```python
from build123d import *

# Parameters (mm, degrees)
SKETCH_1_W          = 72
SKETCH_1_H          = 16
SKETCH_1_R          = 3.1
EXTRUDE_1_DEPTH     = 4
EXTRUDE_START       = -4
SKETCH_3_W          = 30
SKETCH_3_H          = 5
EXTRUDE_2_DEPTH     = 60
SKETCH_5_W          = 108
SKETCH_5_H          = 11
SKETCH_5_R          = 2.1
EXTRUDE_3_DEPTH     = 5
SKETCH_6_W          = 12
SKETCH_6_H          = 11
CUT_EXTRUDE_1_DEPTH = 2
SKETCH_7_W          = 15
SKETCH_7_H          = 50
CUT_EXTRUDE_2_DEPTH = 86.599357474
EXTRUDE_4_DEPTH     = 2
EXTRUDE_START_2     = -30
EXTRUDE_5_DEPTH     = 2
FILLET_1_R          = 2


with BuildPart() as part:
    # 草图1 → 凸台-拉伸1 (new body)
    with BuildSketch(Plane.XY):
        Rectangle(SKETCH_1_W, SKETCH_1_H)
        with Locations((-27.5, 0)):
            Circle(SKETCH_1_R, mode=Mode.SUBTRACT)
        with Locations(Location((27.5, 0, 0), (0, 0, 180))):
            Circle(SKETCH_1_R, mode=Mode.SUBTRACT)
    extrude(amount=EXTRUDE_1_DEPTH)

    # 草图3 → 凸台-拉伸2 (add)
    with BuildSketch(Plane.XY.offset(4).offset(EXTRUDE_START)):
        with Locations((0, -5.5)):
            Rectangle(SKETCH_3_W, SKETCH_3_H)
    extrude(amount=EXTRUDE_2_DEPTH)

    # 草图5 → 凸台-拉伸3 (add, through all)
    with BuildSketch(Plane(origin=(0, -3, 0), x_dir=(1, 0, 0), z_dir=(0, 1, 0))):
        with Locations((0, -60)):
            Rectangle(SKETCH_5_W, SKETCH_5_H)
        with Locations(Location((47.5, -60, 0), (0, 0, 270))):
            Circle(SKETCH_5_R, mode=Mode.SUBTRACT)
        with Locations(Location((-47.5, -60, 0), (0, 0, 90))):
            Circle(SKETCH_5_R, mode=Mode.SUBTRACT)
    extrude(amount=-EXTRUDE_3_DEPTH)

    # 草图6 → 切除-拉伸1 (cut)
    with BuildSketch(Plane(origin=(0, -3, 0), x_dir=(1, 0, 0), z_dir=(0, 1, 0))):
        with Locations((-48, -60)):
            Rectangle(SKETCH_6_W, SKETCH_6_H)
        with Locations((48, -60)):
            Rectangle(SKETCH_6_W, SKETCH_6_H)
    extrude(amount=-CUT_EXTRUDE_1_DEPTH, mode=Mode.SUBTRACT)

    # 草图7 → 切除-拉伸2 (cut, through all)
    with BuildSketch(Plane(origin=(0, -3, 0), x_dir=(1, 0, 0), z_dir=(0, 1, 0))):
        with Locations((0, -34)):
            Rectangle(SKETCH_7_W, SKETCH_7_H)
    extrude(amount=-CUT_EXTRUDE_2_DEPTH, mode=Mode.SUBTRACT)

    # 草图8 → 凸台-拉伸4 (add)
    with BuildSketch(Plane.ZY.offset(15)):
        Polygon((4, -3), (29.25, -3), (4, 8), align=None)
    extrude(amount=-EXTRUDE_4_DEPTH)

    # 草图8<2> → 凸台-拉伸5 (add)
    with BuildSketch(Plane.ZY.offset(15).offset(EXTRUDE_START_2)):
        Polygon((4, -3), (29.25, -3), (4, 8), align=None)
    extrude(amount=EXTRUDE_5_DEPTH)

    # 圆角1
    fillet_1_edges = [part.edges().sort_by_distance(p)[0] for p in [
        (15, 0, 4),
        (36, 0, 4),
        (36, 0, 0),
        (-36, 0, 0),
        (-36, 0, 4),
        (-15, -5.5, 54.5),
        (-54, -6.5, 54.5),
        (-54, -6.5, 65.5),
        (54, -6.5, 65.5),
        (54, -6.5, 54.5),
        (15, -5.5, 54.5),
        (-15, 0, 4),
        (-42, -4, 54.5),
        (42, -4, 54.5),
        (42, -4, 65.5),
        (-42, -4, 65.5),
        (-7.5, -5.5, 59),
        (-7.5, -5.5, 9),
        (7.5, -5.5, 59),
        (7.5, -5.5, 9),
        (14, -3, 29.25),
        (-14, -3, 29.25),
        (-13, 2.5, 4),
        (13, 2.5, 4),
    ]]
    fillet(fillet_1_edges, radius=FILLET_1_R - 0.0001)  # a hair under: the kernel refuses the full size


solid = part.part
```
Geometry check sheet. Reference: the model listing, model coordinates, mm. A direction names the side the tool comes from. Coordinates: 2 decimals unless noted, no trailing zeros. Write each loop counter-clockwise with the first axis right and the second up, starting at its lowest first coordinate (ties: lowest second). Pieces come first, ordered by that corner, then holes. Notation, with made-up numbers: (-33, -25.75) -> (-2, -25.75) arc R12 ccw to (-2, -10.75) -> close; hole circle Ø4 at (33, -33.5). An arc over 180 degrees is marked (long way). Use CSV: the item, a comma, the result in double quotes. Start each with the question number.
Item 1: Cross-section at A-A, the plane x = 47.5. Record the cut outline in (y, z).
Item 2: Cross-section at C-C, the plane z = 14.5. Record the cut outline in (x, y), plus the area to 3 significant figures.
Item 3: Cross-section at B-B, the plane x = 27.5. Record the cut outline in (y, z), plus the area to 3 significant figures.
Item 4: Set-up check for faces 1 (the flat face through (7.5, -5, 34)), 2 (the cylindrical face through (15.6, 0.11, 4.57)), 3 (the flat face through (0, 3, 4)), 4 (the cylindrical face through (-35.43, 0.11, 3.4)): record each of +Z, -Z, +X, -X, +Y, -Y from which the full face is reachable in a straight line by a thin tool's end or side.
Item 5: Cross-section at D-D, the plane x = -22.5. Record the cut outline in (y, z), plus the area to 3 significant figures.
Item 6: Mould release check, pull along Z, two halves, no side actions. Record for faces 5 (the flat face through (30, -5, 54.5)), 6 (the cylindrical face through (12.43, 2.42, 4.6)), 7 (the flat face through (-13, 0, 12)): released by +Z, released by -Z, zero draft, split by the parting line, or undercut.
Item 7: Depth check by flat-ended pin: pin 1 Ø5 at (x, z) = (47.5, 60) entering from +Y; pin 2 Ø1.5 at (x, y) = (37, -5) entering from -Z; pin 3 Ø1.5 at (x, y) = (-1.5, -1.5) entering from +Z. Enter the tip coordinate at first touch or a pass-through.
Item 8: Thickness scan on line 1 (X direction, y = -0.75, z = 23.5); line 2 (Z direction, x = -31, y = -4.25); line 3 (X direction, y = -6.25, z = 34.5). Record the ranges inside material, lowest first.
Answers:
1,outline,"(-8, 54.5) -> (-5, 54.5) -> (-5, 57.9) -> (-8, 57.9) -> close; (-8, 62.1) -> (-5, 62.1) -> (-5, 65.5) -> (-8, 65.5) -> close"
2,outline,"(-15, -8) -> (-7.5, -8) -> (-7.5, -3) -> (-13, -3) -> (-13, 3.43) -> (-15, 3.43) -> close; (7.5, -8) -> (15, -8) -> (15, 3.43) -> (13, 3.43) -> (13, -3) -> (7.5, -3) -> close"
2,area,"101 mm^2"
3,outline,"(-8, 0) -> (-3.1, 0) -> (-3.1, 4) -> (-8, 4) -> close; (-8, 54.5) -> (-3, 54.5) -> (-3, 65.5) -> (-8, 65.5) -> close; (3.1, 0) -> (8, 0) -> (8, 4) -> (3.1, 4) -> close"
3,area,"94.2 mm^2"
4,face 1,"+Y, -Y"
4,face 2,"+X, +Y, -Y"
4,face 3,"+Z, +Y"
4,face 4,"-X, +Y, -Y"
5,outline,"(-8, 0) -> (8, 0) -> (8, 4) -> (-8, 4) -> close; (-8, 54.5) -> (-3, 54.5) -> (-3, 65.5) -> (-8, 65.5) -> close"
5,area,"119 mm^2"
6,face 5,"undercut"
6,face 6,"released by +Z"
6,face 7,"zero draft"
7,pin 1,"y = -5"
7,pin 2,"z = 54.5"
7,pin 3,"z = 4"
8,line 1,"-15 to -13, 13 to 15"
8,line 2,"0 to 4, 54.5 to 65.5"
8,line 3,"-15 to -7.5, 7.5 to 15"
